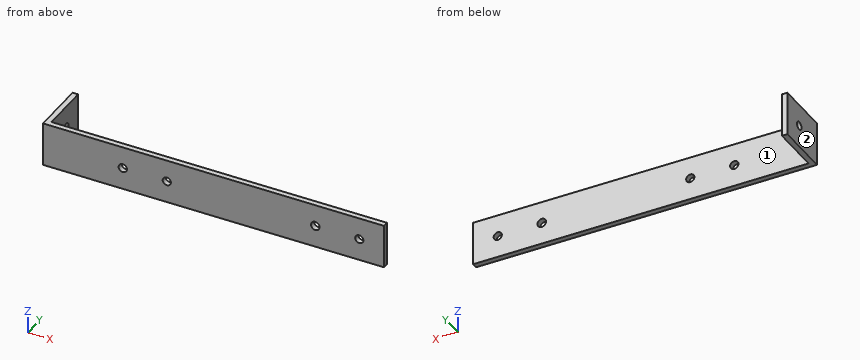
```python
from build123d import *

# Parameters (mm, degrees)
F1_DEPTH = 25.4
F2_R     = 4.7625
F3_DEPTH = 6.351
F4_R     = 4.739103
F4_R_2   = 5.002197
F4_R_3   = 4.826
F5_DEPTH = 6.351


with BuildPart() as f1:
    # F0 (on Top) → F1 (new body, symmetric)
    with BuildSketch(Plane.XY):
        Polygon((0, 0), (393.7, 0), (393.7, 6.35), (6.35, 6.35), (6.35, 63.5), (0, 63.5), align=None)
    extrude(amount=F1_DEPTH, both=True)

    # F2 (on face) → F3 (cut, through all)
    with BuildSketch(Plane.YZ.offset(6.35)):
        with Locations((38.1, 0)):
            Circle(F2_R)
    extrude(amount=-F3_DEPTH, mode=Mode.SUBTRACT)

    # F4 (on face) → F5 (cut, through all)
    with BuildSketch(Plane(origin=(0, 6.35, 0), x_dir=(-1, 0, 0), z_dir=(0, 1, 0))):
        with Locations((-365.125, 0)):
            Circle(F4_R)
        with Locations((-314.325, 0)):
            Circle(F4_R_2)
        with Locations((-142.875, 0)):
            Circle(F4_R)
        with Locations((-92.075, 0)):
            Circle(F4_R_3)
    extrude(amount=-F5_DEPTH, mode=Mode.SUBTRACT)


solid = f1.part
```
CAD build for the part. Positions are in the model's coordinates, mm. Face numbers are marked on the shaded views. A direction names the side the tool comes from. Round coordinates to 2 decimals unless told otherwise and drop trailing zeros. Write each loop counter-clockwise with the first axis right and the second up, starting at its lowest first coordinate (ties: lowest second). Pieces come first, ordered by that corner, then holes. Notation, with made-up numbers: (88, -39) - (137, -39) arc R10 cw to (137, -31) - close; hole circle Ø6 at (-9.75, -13). An arc over 180 degrees is marked (long way). Return JSON: item names as keys, results as strings. Group by question number.
Item 1: Band-saw the part on D-D on z = -19. List the corners of the cut face in (x, y).
Item 2: Band-saw the part on A-A on z = 0. List the corners of the cut face in (x, y), plus the area to 3 significant figures.
Item 3: 3-axis set-ups, long thin cutter, end or side, ignore diameter. For the marked faces 1 and 2: which of +Z, -Z, +X, -X, +Y, -Y reach the whole face in a straight line?
Item 4: Band-saw the part on C-C on x = 194. List the corners of the cut face in (y, z).
Item 5: Band-saw the part on B-B on y = 38.1. List the corners of the cut face in (x, z), plus the area to 3 significant figures.
Item 6: Flat gauge pins, fed straight in: pin 1 Ø6 at (y, z) = (37, -13) entering from -X; pin 2 Ø15 at (x, z) = (197.5, 4.5) entering from +Y. Where does each tip first touch, or does it go through?
Item 7: Probe probe 1 along Z at (x, y) = (4, 38.1); probe 2 along Y at (x, z) = (104, -17). List the from-to ranges inside material, lowest first.
Resolved:
{
 "1": {"outline": "(0, 0) - (393.7, 0) - (393.7, 6.35) - (6.35, 6.35) - (6.35, 63.5) - (0, 63.5) - close"},
 "2": {"outline": "(0, 0) - (87.25, 0) - (87.25, 6.35) - (6.35, 6.35) - (6.35, 33.34) - (0, 33.34) - close; (0, 42.86) - (6.35, 42.86) - (6.35, 63.5) - (0, 63.5) - close; (96.9, 0) - (138.14, 0) - (138.14, 6.35) - (96.9, 6.35) - close; (147.61, 0) - (309.32, 0) - (309.32, 6.35) - (147.61, 6.35) - close; (319.33, 0) - (360.39, 0) - (360.39, 6.35) - (319.33, 6.35) - close; (369.86, 0) - (393.7, 0) - (393.7, 6.35) - (369.86, 6.35) - close", "area": "2,560 mm²"},
 "3": {"face 1": "+Z, -Z, +X, +Y", "face 2": "+Z, -Z, -X, +Y, -Y"},
 "4": {"outline": "(0, -25.4) - (6.35, -25.4) - (6.35, 25.4) - (0, 25.4) - close"},
 "5": {"outline": "(0, -25.4) - (6.35, -25.4) - (6.35, -4.76) - (0, -4.76) - close; (0, 4.76) - (6.35, 4.76) - (6.35, 25.4) - (0, 25.4) - close", "area": "262 mm²"},
 "6": {"pin 1": "stops at x = 0", "pin 2": "stops at y = 6.35"},
 "7": {"probe 1": "z = -25.4 to -4.76, 4.76 to 25.4", "probe 2": "y = 0 to 6.35"}
}
